```python
from build123d import *

# Parameters (mm, degrees)
SKETCH3_W          = 6.35
SKETCH3_H          = 6.35
CUT_EXTRUDE2_DEPTH = 16.476293161
SKETCH4_R          = 5.207
CUT_EXTRUDE3_DEPTH = 1.143
FILLET1_R          = 0.635
FILLET2_R          = 7.62


with BuildPart() as part:
    # Sketch1 → Revolve1 (revolve)
    with BuildSketch(Plane.XY, mode=Mode.PRIVATE) as revolve1_sk:
        with BuildLine():
            Line((8.255, -2.54), (8.255, -5.08))
            Line((8.255, -5.08), (0, -5.08))
            Line((0, -5.08), (0, 5.08))
            Line((0, 5.08), (8.255, 5.08))
            Line((8.255, 5.08), (8.255, 2.54))
            ThreePointArc((8.255, 2.54), (5.715, 0), (8.255, -2.54))
        make_face()
    revolve(revolve1_sk.sketch.rotate(Axis((0, -5.08, 0), (0, 1, 0)), 90), axis=Axis((0, -5.08, 0), (0, 1, 0)))

    # Sketch3 → Cut-Extrude2 (cut, through all)
    with BuildSketch(Plane(origin=(0, 5.08, 0), x_dir=(1, 0, 0), z_dir=(0, 1, 0))):
        Rectangle(SKETCH3_W, SKETCH3_H)
    extrude(amount=-CUT_EXTRUDE2_DEPTH, mode=Mode.SUBTRACT)

    # Sketch4 → Cut-Extrude3 (cut)
    with BuildSketch(Plane(origin=(0, 5.08, 0), x_dir=(1, 0, 0), z_dir=(0, 1, 0))):
        with Locations(Location((0, 0, 0), (0, 0, 270))):
            Circle(SKETCH4_R)
    cut_extrude3 = extrude(amount=-CUT_EXTRUDE3_DEPTH, mode=Mode.SUBTRACT)

    # Mirror1: Cut-Extrude3 across plane
    add(cut_extrude3.mirror(Plane.ZX), mode=Mode.SUBTRACT)

    # Fillet1
    fillet1_edges = [part.edges().sort_by_distance(p)[0] for p in [
        (0, 5.08, 8.255),
        (0, -5.08, 8.255),
    ]]
    fillet(fillet1_edges, radius=FILLET1_R)

    # Fillet2
    # the kernel refuses this fillet: 7.62 mm, written as the material it takes off along each edge
    with BuildSketch(Plane(origin=(0, 2.54, 0), x_dir=(0, 0, -1), z_dir=(1, 0, 0))) as fillet2_piece_1:
        with BuildLine():
            CenterArc((1.191070941, 4.7625), FILLET2_R, 314.048625674, 23.927061489)
            Line((8.255, 1.905), (8.396278581, 1.84785))
            ThreePointArc((8.396278581, 1.84785), (8.4074, 0.9525), (8.4074, 0))
            Line((8.4074, 0), (8.255, -0.1524))
            ThreePointArc((8.255, -0.1524), (7.35965, -0.326635562), (6.594976671, -0.8239125))
            Line((6.594976671, -0.8239125), (6.489017735, -0.714375))
        make_face()
    revolve(axis=Axis((0, 2.54, 0), (0, 1, 0)), mode=Mode.SUBTRACT)
    with BuildSketch(Plane(origin=(0, -2.54, 0), x_dir=(0, 0, -1), z_dir=(1, 0, 0))) as fillet2_piece_2:
        with BuildLine():
            CenterArc((1.191070941, -4.7625), FILLET2_R, 22.024312837, 23.927061489)
            Line((6.489017735, 0.714375), (6.594976671, 0.8239125))
            ThreePointArc((6.594976671, 0.8239125), (7.35965, 0.326635562), (8.255, 0.1524))
            Line((8.255, 0.1524), (8.4074, 0))
            ThreePointArc((8.4074, 0), (8.4074, -0.9525), (8.396278581, -1.84785))
            Line((8.396278581, -1.84785), (8.255, -1.905))
        make_face()
    revolve(axis=Axis((0, -2.54, 0), (0, 1, 0)), mode=Mode.SUBTRACT)


solid = part.part
```
Work out the finished part from the listing and answer in its coordinate system (mm). A direction names the side the tool comes from. Give positions to 0.01 mm unless a question says otherwise; leave off trailing zeros. Loops run counter-clockwise (first coordinate to the right, second up) from the corner with the lowest first, then second, coordinate; pieces in that order, holes last. Notation, with made-up numbers: (62.25, 20.5) -> (94.25, 20.5) arc R29 cw to (94.25, 44.5) -> close; hole circle Ø6 at (83.25, 42.25). An arc over 180 degrees is marked (long way). Use CSV: the item, a comma, the result in double quotes.
1. The part is cut by section B-B (y = 1.5). Write down the section's boundary in (x, z) (3 decimals).
Found:
outline,"circle Ø12.41 at (0, 0); hole (-3.175, -3.175) -> (3.175, -3.175) -> (3.175, 3.175) -> (-3.175, 3.175) -> close"
2. Flat-ended cylindrical pins translate along their axes: pin 1 Ø3 at (x, z) = (-0.5, -2) entering from +Y; pin 2 Ø5 at (x, y) = (0, 1) entering from +Z; pin 3 Ø1.5 at (y, z) = (0.5, -4) entering from +X. Find the tip coordinate at first contact, or state that the pin passes through.
Found:
pin 1,"y = 3.94"
pin 2,"z = 7.79"
pin 3,"x = 4.82"
3. Straight lines are drawn through the part: line 1 (X direction, y = -4.5, z = 0); line 2 (Z direction, x = -1.75, y = 1.25) (3 decimals). For each, find the intervals that lie inside material, in ascending order.
Found:
line 1,"-8.25 to -5.21, 5.21 to 8.25"
line 2,"-5.785 to -3.175, 3.175 to 5.785"
4. The part is cut by section A-A (y = -1.25). Write down the section's boundary in (x, z) (3 decimals), then the cut area to 3 significant figures.
Found:
outline,"circle Ø12.088 at (0, 0); hole (-3.175, -3.175) -> (3.175, -3.175) -> (3.175, 3.175) -> (-3.175, 3.175) -> close"
area,"74.4 mm^2"
5. A tool of negligible diameter and unlimited length cuts with its end or side. For faces 3 (the flat face through (2, 5.08, 5)), 4 (the flat face through (0, 0, -3.175)), 5 (the flat face through (-3.4, 3.937, -0.1)), 6 (the flat face through (-3.4, -3.937, -0.1)), from which of +Z, -Z, +X, -X, +Y, -Y can it reach the whole face along a straight path? Write none if from no direction.
Found:
face 3,"+Z, -Z, +X, -X, +Y"
face 4,"+Y, -Y"
face 5,"+Y"
face 6,"-Y"
6. The mould has two halves that part along Z. Classify faces 1 (the flat face through (5, -5.08, -2)), 2 (the flat face through (0, 0, 3.175)): +Z half, -Z half, draft (parallel to the pull), parting line (faces both ways), or undercut.
Found:
face 1,"draft"
face 2,"undercut"
